Part model, mm, in its own coordinate system. Give positions to 0.01 mm unless a question says otherwise; leave off trailing zeros. Write each loop counter-clockwise with the first axis right and the second up, starting at its lowest first coordinate (ties: lowest second). Pieces come first, ordered by that corner, then holes. Notation, with made-up numbers: M -21,75.25 L 7,75.25 A18 ccw 7,100.25 Z; hole C 63.5,-30 d9. An arc over 180 degrees is marked long. Answer as CSV lines item,"result". Start each with the question number.
1) Slice it at A-A, the plane y = 1. Give the cut face in (x, z), plus the area to 3 significant figures.
2) Slice it at B-B, the plane x = 18. Give the cut face in (y, z), plus the area to 3 significant figures.
3) Slice it at C-C, the plane z = -115. Give the cut face in (x, y).
4) Wall check: line 1 along X through (y, z) = (0.6, -11); line 2 along Z through (x, y) = (10, 0.55); line 3 along X through (y, z) = (0.4, -6) (3 decimals). Give the ranges that are in metal, low to high. Write a range as from..to.
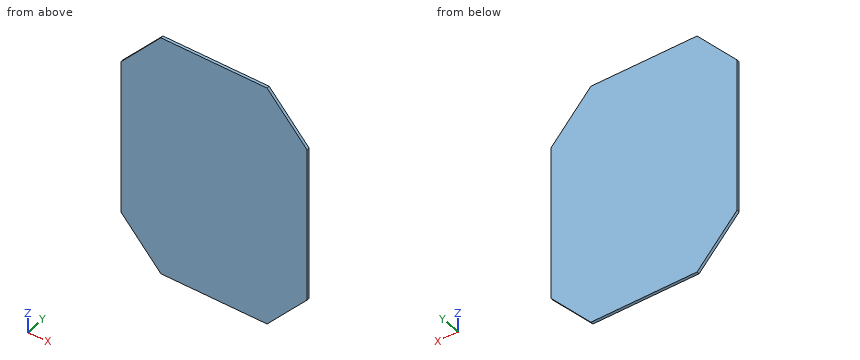
```python
from build123d import *

# Parameters (mm, degrees)
SKETCH1_W           = 100
SKETCH1_H           = 132
BOSS_EXTRUDE1_DEPTH = 1.5
CUT_EXTRUDE1_DEPTH  = 1.5


with BuildPart() as part:
    # Sketch1 → Boss-Extrude1 (new body)
    with BuildSketch(Plane(origin=(0, 0, 0), x_dir=(1, 0, 0), z_dir=(0, 1, 0))):
        with Locations((50, 66)):
            Rectangle(SKETCH1_W, SKETCH1_H)
    extrude(amount=BOSS_EXTRUDE1_DEPTH)

    # Sketch2 → Cut-Extrude1 (cut)
    with BuildSketch(Plane(origin=(0, 1.5, 0), x_dir=(1, 0, 0), z_dir=(0, 1, 0))):
        Polygon((78.5, 132), (100, 108), (126.790697674, 132), (105.290697674, 156), align=None)
        Polygon((-26.790697674, 132), (-5.290697674, 156), (21.5, 132), (0, 108), align=None)
        Polygon((126.790697674, 0), (105.290697674, -24), (78.5, 0), (100, 24), align=None)
        Polygon((0, 24), (-26.790697674, 0), (-5.290697674, -24), (21.5, 0), align=None)
    extrude(amount=-CUT_EXTRUDE1_DEPTH, mode=Mode.SUBTRACT)


solid = part.part
```
Found:
1,outline,"M 0,-108 L 21.5,-132 L 78.5,-132 L 100,-108 L 100,-24 L 78.5,0 L 21.5,0 L 0,-24 Z"
1,area,"12,200 mm²"
2,outline,"M 0,-128.09 L 1.5,-128.09 L 1.5,-3.91 L 0,-3.91 Z"
2,area,"186 mm²"
3,outline,"M 6.27,0 L 93.73,0 L 93.73,1.5 L 6.27,1.5 Z"
4,line 1,"11.65..88.35"
4,line 2,"-119.16..-12.84"
4,line 3,"16.125..83.875"
